Design review of the part built by this model. Coordinates are the model's own, in mm. A direction names the side the tool comes from. Round coordinates to 2 decimals unless told otherwise and drop trailing zeros. Order: outer loops, then holes, each group sorted by start corner. A loop starts at its lowest first (then second) coordinate and runs counter-clockwise, first axis right, second up. Notation, with made-up numbers: (-24, -31.75) - (12, -31.75) arc R21 ccw to (12, -10.75) - close; hole circle Ø8 at (-0.75, 61). An arc over 180 degrees is marked (long way). Use CSV: the item, a comma, the result in double quotes.
from build123d import *

# Parameters (mm, degrees)
F0_W     = 60
F0_H     = 50
F1_DEPTH = 13
F3_DEPTH = 60
F4_R     = 3.25
F5_DEPTH = 50
F6_R     = 2.5
F7_DEPTH = 10


with BuildPart() as f1:
    # F0 (on Top) → F1 (new body, symmetric)
    with BuildSketch(Plane.XY):
        Rectangle(F0_W, F0_H)
    extrude(amount=F1_DEPTH, both=True)

    # F2 (on face) → F3 (cut)
    with BuildSketch(Plane.YZ.offset(30)):
        Polygon((-11.055123, 13), (-14.538462, 0), (25, 0), (25, 13), align=None)
    extrude(amount=-F3_DEPTH, mode=Mode.SUBTRACT)

    # F4 (on face) → F5 (cut)
    with BuildSketch(Plane(origin=(0, 25, 0), x_dir=(-1, 0, 0), z_dir=(0, 1, 0))):
        with Locations((0, -6.5)):
            Circle(F4_R)
    extrude(amount=-F5_DEPTH, mode=Mode.SUBTRACT)

    # F6 (on face) → F7 (cut)
    with BuildSketch(Plane(origin=(0, 25, 0), x_dir=(-1, 0, 0), z_dir=(0, 1, 0))):
        with Locations((-20, -6.5)):
            Circle(F6_R)
        with Locations((20, -6.5)):
            Circle(F6_R)
    extrude(amount=-F7_DEPTH, mode=Mode.SUBTRACT)


solid = f1.part
1) We need section A-A (y = 16). Give the boundary of the cut face in (x, z).
Data:
outline,"(-30, -13) - (30, -13) - (30, 0) - (-30, 0) - close; hole circle Ø5 at (-20, -6.5); hole circle Ø6.5 at (0, -6.5); hole circle Ø5 at (20, -6.5)"
2) Insertion check: pin 1 Ø8 at (x, z) = (13, 6) entering from +Y; pin 2 Ø20 at (x, y) = (10.5, 8) entering from +Z; pin 3 Ø5.5 at (x, z) = (-20, -7) entering from +Y; pin 4 Ø4.5 at (x, z) = (-20, -6.5) entering from +Y. Each pin has a flat end and moves straight along its axis. Give the tip position at first contact, or say it passes through.
Data:
pin 1,"stops at y = -11.86"
pin 2,"stops at z = 0"
pin 3,"stops at y = 25"
pin 4,"stops at y = 15"
3) To check wall thickness, follow L1, parallel to Z at x = -20, y = 18; L2, parallel to Z at x = 17, y = 8; L3, parallel to X at y = 8.5, z = -4.25. State the ranges of each line that lie inside material, in increasing order. Write a range as from..to.
Data:
L1,"z = -13..-9, -4..0"
L2,"z = -13..0"
L3,"x = -30..-2.35, 2.35..30"
4) We need section D-D (x = 20). Give the boundary of the cut face in (y, z), then the cut area to 3 significant figures.
Data:
outline,"(-25, -13) - (25, -13) - (25, -9) - (15, -9) - (15, -4) - (25, -4) - (25, 0) - (-14.54, 0) - (-11.06, 13) - (-25, 13) - close"
area,"759 mm2"
5) We need section C-C (x = 0). Give the boundary of the cut face in (y, z), then the cut area to 3 significant figures.
Data:
outline,"(-25, -13) - (25, -13) - (25, -9.75) - (-25, -9.75) - close; (-25, -3.25) - (25, -3.25) - (25, 0) - (-14.54, 0) - (-11.06, 13) - (-25, 13) - close"
area,"484 mm2"
6) For faces 1 (the face through (0.42, -12.772, 6.591)), 2 (the face through (-20, 15, -6)), 3 (the face through (-30, -6, -3)), list the 3-axis set-ups (+Z, -Z, +X, -X, +Y, -Y) from which the entire face can be reached by the end or side of a thin tool; tool diameter is ignored.
Data:
face 1,"+X, -X, +Y"
face 2,"+Y"
face 3,"+Z, -Z, -X, +Y, -Y"
7) We need section B-B (z = -6.5). Give the boundary of the cut face in (x, y).
Data:
outline,"(-30, -25) - (-3.25, -25) - (-3.25, 25) - (-17.5, 25) - (-17.5, 15) - (-22.5, 15) - (-22.5, 25) - (-30, 25) - close; (3.25, -25) - (30, -25) - (30, 25) - (22.5, 25) - (22.5, 15) - (17.5, 15) - (17.5, 25) - (3.25, 25) - close"
